The listing builds one solid part. Answer for the finished solid, in the listing's coordinates (mm). A direction names the side the tool comes from. Coordinates: 2 decimals unless noted, no trailing zeros. Order: outer loops, then holes, each group sorted by start corner. A loop starts at its lowest first (then second) coordinate and runs counter-clockwise, first axis right, second up. Notation, with made-up numbers: (48.5, 32) -> (78.5, 32) arc R16 ccw to (78.5, 54) -> close; hole circle Ø10 at (83.25, 55). An arc over 180 degrees is marked (long way). Answer in a Markdown table with one row per item.
```python
from build123d import *

# Parameters (mm, degrees)
F1_DEPTH = 40
F2_R     = 19.99999
F3_R     = 10
F4_DEPTH = 12.001


# Not quite as in the source:
# - a fillet or chamfer is up to 0.001 mm smaller than in the source, because OpenCascade refuses the exact size


with BuildPart() as f1:
    # F0 (on Front) → F1 (new body)
    with BuildSketch(Plane.XZ):
        Polygon((0, 20), (0, 0), (75, 0), (75, 10), (50, 10), (50, 20), (40, 20), (40, 12), (10, 12), (10, 20), align=None)
    extrude(amount=F1_DEPTH)

    # F2 (radius 20 in the source; OpenCascade refuses exactly that, so slightly less here)
    f2_edges = [f1.edges().sort_by_distance(p)[0] for p in [
        (75, -40, 5),
        (75, 0, 5),
    ]]
    fillet(f2_edges, radius=F2_R)

    # F3 (on face) → F4 (cut, through all)
    with BuildSketch(Plane.XY.offset(12)):
        with Locations((25, -20)):
            Circle(F3_R)
    extrude(amount=-F4_DEPTH, mode=Mode.SUBTRACT)


solid = f1.part
```
(1) A cutting plane is placed at C-C, the plane y = -18. Determine the outline of the cut face in (x, z), then the cut area to 3 significant figures.
Check values:
| item | result |
|---|---|
| outline | (0, 0) -> (15.2, 0) -> (15.2, 12) -> (10, 12) -> (10, 20) -> (0, 20) -> close; (34.8, 0) -> (74.9, 0) -> (74.9, 10) -> (50, 10) -> (50, 20) -> (40, 20) -> (40, 12) -> (34.8, 12) -> close |
| area | 774 mm² |
(2) For a pull along X with two mould halves and no side action, classify faces 4 (the cylindrical face through (69.297, -33.986, 5.07)), 5 (the flat face through (10, -20, 16)), 6 (the flat face through (0, -20, 10)), 7 (the flat face through (27, -40, 8)) as released by +X, released by -X, zero draft, split by the parting line, or undercut.
Check values:
| item | result |
|---|---|
| face 4 | released by +X |
| face 5 | undercut |
| face 6 | released by -X |
| face 7 | zero draft |
(3) A cutting plane is placed at B-B, the plane x = 25. Determine the outline of the cut face in (y, z), then the cut area to 3 significant figures.
Check values:
| item | result |
|---|---|
| outline | (-40, 0) -> (-30, 0) -> (-30, 12) -> (-40, 12) -> close; (-10, 0) -> (0, 0) -> (0, 12) -> (-10, 12) -> close |
| area | 240 mm² |
(4) Which of the six approach directions +Z, -Z, +X, -X, +Y, -Y give full straight-line access (tool end or side, diameter ignored) to faces 1 (the flat face through (50, -20, 15)), 2 (the flat face through (45, -20, 20)), 3 (the flat face through (40, -20, 16))?
Check values:
| item | result |
|---|---|
| face 1 | +Z, +X, +Y, -Y |
| face 2 | +Z, +X, -X, +Y, -Y |
| face 3 | +Z, +Y, -Y |
(5) Find the intervals of material crossed by line 1 along Y through (x, z) = (25, 3.75); line 2 along X through (y, z) = (-9, 12.75); line 3 along Z through (x, y) = (25.5, -34), in increasing order. Write a range as from..to.
Check values:
| item | result |
|---|---|
| line 1 | -40..-30, -10..0 |
| line 2 | 0..10, 40..50 |
| line 3 | 0..12 |
(6) A cutting plane is placed at A-A, the plane z = 14.5. Determine the outline of the cut face in (x, y).
Check values:
| item | result |
|---|---|
| outline | (0, -40) -> (10, -40) -> (10, 0) -> (0, 0) -> close; (40, -40) -> (50, -40) -> (50, 0) -> (40, 0) -> close |
(7) Flat-ended cylindrical pins translate along their axes: pin 1 (2 mm diameter, centred on y = -17.5, z = 9, fed in from +X); pin 2 (11 mm diameter, centred on y = -26.5, z = 16, fed in from +X); pin 3 (10 mm diameter, centred on x = 20, y = -27, fed in from +Z). Find the tip coordinate at first contact, or state that the pin passes through.
Check values:
| item | result |
|---|---|
| pin 1 | x = 74.94 |
| pin 2 | x = 50 |
| pin 3 | z = 12 |
